Autodesk Inventor part; units mm, degrees
ref_plane "YZ Plane" through (0, 0, 0) normal (1, 0, 0) x (0, 1, 0)
ref_plane "XZ Plane" through (0, 0, 0) normal (0, 1, 0) x (-1, 0, 0)
ref_plane "XY Plane" through (0, 0, 0) normal (0, 0, 1) x (1, 0, 0)
sketch "Sketch1" plane through (0, 0, 0) normal (0, 0, 1) x (1, 0, 0)
  line L0 (-36, 20) -> (36, 20)
  line L1 (36, 20) -> (36, -20)
  line L2 (36, -20) -> (-36, -20)
  line L3 (-36, -20) -> (-36, 20)
  line L4 (-36, 20) -> (36, -20) construction
  line L5 (36, 20) -> (-36, -20) construction
  point P0 (0, 0)
  dimension "d0" = 40
  dimension "d1" = 72
sketch "Sketch2" plane through (0, 0, 1) normal (0, 0, 1) x (1, 0, 0)
  line L0 (-36, 20) -> (36, 20)
  line L1 (-46, -5) -> (-36, -5)
  line L2 (-36, -5) -> (-36, 5)
  line L3 (-36, 5) -> (-46, 5)
  line L4 (-46, 5) -> (-46, -5)
  line L5 (-46, -5) -> (-36, 5) construction
  line L6 (-36, -5) -> (-46, 5) construction
  line L7 (0, 0) -> (0, 7.0571)
  line L8 (0, 0) -> (6.6312, 0)
  line L9 (-36, -20) -> (-36, 20)
  line L10 (46, -5) -> (36, -5)
  line L11 (36, -5) -> (36, 5)
  line L12 (36, 5) -> (46, 5)
  line L13 (46, 5) -> (46, -5)
  line L14 (46, -5) -> (36, 5) construction
  line L15 (36, -5) -> (46, 5) construction
  circle A0 centre (-42, 0) radius 1.6
  circle A1 centre (42, 0) radius 1.6
  line L16 (36, -20) -> (-36, -20)
  line L17 (-5, -30) -> (5, -30)
  line L18 (5, -30) -> (5, -20)
  line L19 (5, -20) -> (-5, -20)
  line L20 (-5, -20) -> (-5, -30)
  line L21 (-5, -30) -> (5, -20) construction
  line L22 (5, -30) -> (-5, -20) construction
  circle A2 centre (0, -26) radius 1.6
  line L23 (-5, 30) -> (5, 30)
  line L24 (5, 30) -> (5, 20)
  line L25 (5, 20) -> (-5, 20)
  line L26 (-5, 20) -> (-5, 30)
  line L27 (-5, 30) -> (5, 20) construction
  line L28 (5, 30) -> (-5, 20) construction
  circle A3 centre (0, 26) radius 1.6
  point P0 (-41, 0)
  point P1 (41, 0)
  point P2 (0, -25)
  point P3 (0, 25)
  dimension "d5" = 10
  dimension "d6" = 10
  dimension "d10" = 3.2
  dimension "d12" = 4
  dimension "d18" = 3.2
  dimension "d19" = 10
  dimension "d20" = 10
  dimension "d21" = 4
extrude "Plate1" add sketch "Sketch1" along normal blind 1
sheet face with bend "Face2" sketch "Sketch2" thickness 1 toward (0, 0, -1) bend radius 1
bend "Bend1"
equation "\"d2\" = 厚度"
equation "\"d13\" = 折彎半徑"
equation "\"d14\" = 折彎離隙寬度"
equation "\"d16\" = 最小剩餘"
equation "\"d15\" = 折彎離隙深度"
equation "\"d17\" = 轉移半徑"
equation "\"折彎半徑\" = 厚度"
equation "\"折彎離隙寬度\" = 厚度"
equation "\"折彎離隙深度\" = 0.5 * 厚度"
equation "\"轉角離隙大小\" = 4 * 厚度"
equation "\"最小剩餘\" = 2 * 厚度"
equation "\"轉移半徑\" = 折彎半徑"
equation "\"Jacobi半徑大小\" = 折彎半徑"
equation "\"間隙大小\" = 厚度"
properties part number "battery_box_5V_base" material "Aluminum"
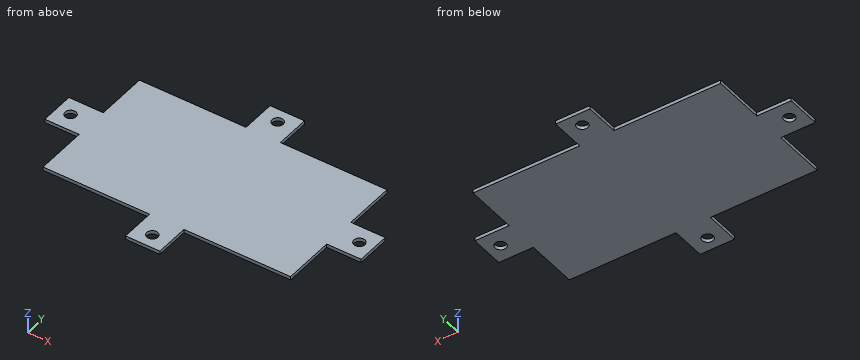
Can you work these out from the model? Positions are in its coordinate system, mm. Give positions to 0.01 mm unless a question says otherwise; leave off trailing zeros. Loops run counter-clockwise (first coordinate to the right, second up) from the corner with the lowest first, then second, coordinate; pieces in that order, holes last. Notation, with made-up numbers: (7.25, -18) - (41.25, -18) arc R12 ccw to (41.25, -12) - close; hole circle Ø9 at (16, 43). An arc over 180 degrees is marked (long way). Return JSON: item names as keys, results as strings.
1. If I drill on line 1 (Y direction, x = 0, z = 0.25); line 2 (Y direction, x = -35, z = 0.25); line 3 (X direction, y = -14.5, z = 0.35), over which ranges is the centre line in solid material (lowest first)?
Output values:
{"line 1": "y = -30 to -27.6, -24.4 to 24.4, 27.6 to 30", "line 2": "y = -20 to 20", "line 3": "x = -36 to 36"}
2. I want a section at C-C on z = 0.8. Please give me the cut outline in (x, y), and give its area (3 significant figures).
Output values:
{"outline": "(-46, -5) - (-36, -5) - (-36, -20) - (-5, -20) - (-5, -30) - (5, -30) - (5, -20) - (36, -20) - (36, -5) - (46, -5) - (46, 5) - (36, 5) - (36, 20) - (5, 20) - (5, 30) - (-5, 30) - (-5, 20) - (-36, 20) - (-36, 5) - (-46, 5) - close; hole circle Ø3.2 at (-42, 0); hole circle Ø3.2 at (0, -26); hole circle Ø3.2 at (0, 26); hole circle Ø3.2 at (42, 0)", "area": "3,250 mm²"}
3. I want a section at D-D on y = 0. Please give me the cut outline in (x, z), and give its area (3 significant figures).
Output values:
{"outline": "(-46, 0) - (-43.6, 0) - (-43.6, 1) - (-46, 1) - close; (-40.4, 0) - (40.4, 0) - (40.4, 1) - (-40.4, 1) - close; (43.6, 0) - (46, 0) - (46, 1) - (43.6, 1) - close", "area": "85.6 mm²"}
4. I want a section at A-A on x = 0. Please give me the cut outline in (y, z).
Output values:
{"outline": "(-30, 0) - (-27.6, 0) - (-27.6, 1) - (-30, 1) - close; (-24.4, 0) - (24.4, 0) - (24.4, 1) - (-24.4, 1) - close; (27.6, 0) - (30, 0) - (30, 1) - (27.6, 1) - close"}
5. I want a section at B-B on y = 26. Please give me the cut outline in (x, z).
Output values:
{"outline": "(-5, 0) - (-1.6, 0) - (-1.6, 1) - (-5, 1) - close; (1.6, 0) - (5, 0) - (5, 1) - (1.6, 1) - close"}
6. I'm going to push flat-ended pins straight in: pin 1 Ø1.9 at (x, y) = (42, 0) entering from -Z; pin 2 Ø0.5 at (y, z) = (-26.5, 0.5) entering from -X; pin 3 Ø0.5 at (x, z) = (39, 0.5) entering from +Y; pin 4 Ø0.5 at (x, z) = (20.5, 0.5) entering from -Y. Where does each tip first touch, or does it pass through?
Output values:
{"pin 1": "passes through", "pin 2": "stops at x = -5", "pin 3": "stops at y = 5", "pin 4": "stops at y = -20"}
